Design review of the part built by this model. Coordinates are the model's own, in mm. Face numbers are marked on the shaded views. Coordinates: 2 decimals unless noted, no trailing zeros. Write each loop counter-clockwise with the first axis right and the second up, starting at its lowest first coordinate (ties: lowest second). Pieces come first, ordered by that corner, then holes.
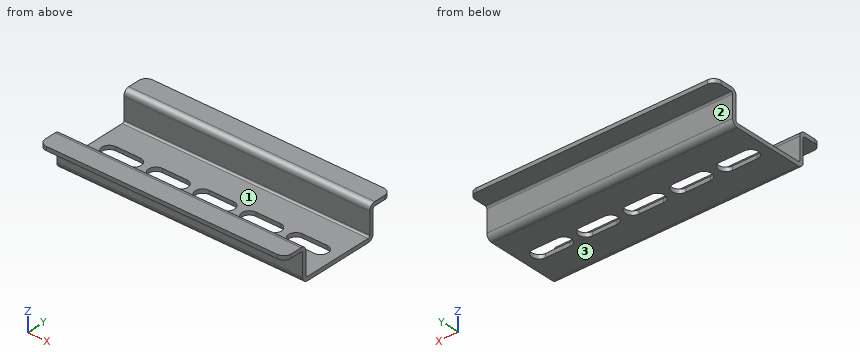
```python
from build123d import *

# Parameters (mm, degrees)
SKETCH_1_W                         = 100
SKETCH_1_H                         = 30
SM_BASE_FLANGE_1_DEPTH             = 1.6
SM_EDGE_FLANGE_1_STRIP_W           = 7.8732
SM_EDGE_FLANGE_1_STRIP_H           = 1.6
SM_EDGE_FLANGE_1_STRIP_CUT_DEPTH   = 100
SM_EDGE_FLANGE_1_STRIP_2_W         = 7.8732
SM_EDGE_FLANGE_1_STRIP_2_H         = 1.6
SM_EDGE_FLANGE_1_STRIP_CUT_2_DEPTH = 100
SM_EDGE_FLANGE_1_DEPTH             = 100
SM_EDGE_FLANGE_1_BEND_DEPTH        = 100
SM_EDGE_FLANGE_2_STRIP_W           = 7.8732
SM_EDGE_FLANGE_2_STRIP_H           = 1.6
SM_EDGE_FLANGE_2_STRIP_CUT_DEPTH   = 100
SM_EDGE_FLANGE_2_STRIP_2_W         = 7.8732
SM_EDGE_FLANGE_2_STRIP_2_H         = 1.6
SM_EDGE_FLANGE_2_STRIP_CUT_2_DEPTH = 100
SM_EDGE_FLANGE_2_DEPTH             = 100
SM_EDGE_FLANGE_2_BEND_DEPTH        = 100
CUT_EXTRUDE_1_DEPTH                = 58.175169436
CUT_EXTRUDE_2_DEPTH                = 58.532251825


# Sheet-metal steps are written as plain solids
with BuildPart() as part:
    # Sketch 1 → 基体-法兰1 (new body)
    with BuildSketch(Plane.XY):
        Rectangle(SKETCH_1_W, SKETCH_1_H)
    extrude(amount=-SM_BASE_FLANGE_1_DEPTH)

    # 边线-法兰1 strip (across the edge) → 边线-法兰1 strip cut (cut)
    with BuildSketch(Plane(origin=(50, 15, 0), x_dir=(0, -1, 0), z_dir=(-1, 0, 0))):
        with Locations((-3.2, -0.8)):
            Rectangle(SM_EDGE_FLANGE_1_STRIP_W, SM_EDGE_FLANGE_1_STRIP_H)
    extrude(amount=SM_EDGE_FLANGE_1_STRIP_CUT_DEPTH, mode=Mode.SUBTRACT)

    # 边线-法兰1 strip 2 (across the edge) → 边线-法兰1 strip cut 2 (cut)
    with BuildSketch(Plane(origin=(-50, -15, 0), x_dir=(0, 1, 0), z_dir=(1, 0, 0))):
        with Locations((-3.2, -0.8)):
            Rectangle(SM_EDGE_FLANGE_1_STRIP_2_W, SM_EDGE_FLANGE_1_STRIP_2_H)
    extrude(amount=SM_EDGE_FLANGE_1_STRIP_CUT_2_DEPTH, mode=Mode.SUBTRACT)

    # 边线-法兰1 section (across the edge) → 边线-法兰1 (add)
    with BuildSketch(Plane(origin=(50, 15, 0), x_dir=(0, -1, 0), z_dir=(-1, 0, 0))):
        with BuildLine():
            Line((-1.6, 0.7366), (-1.6, 10.4))
            Line((-1.6, 10.4), (0, 10.4))
            Line((0, 10.4), (0, 0.7366))
            ThreePointArc((0, 0.7366), (0.215745145, 0.215745145), (0.7366, 0))
            Line((0.7366, 0), (0.7366, -1.6))
            ThreePointArc((0.7366, -1.6), (-0.915625705, -0.915625705), (-1.6, 0.7366))
        make_face()
    extrude(amount=SM_EDGE_FLANGE_1_DEPTH)

    # 边线-法兰1 section 2 (across the edge) → 边线-法兰1 bend (add)
    with BuildSketch(Plane(origin=(-50, -15, 0), x_dir=(0, 1, 0), z_dir=(1, 0, 0))):
        with BuildLine():
            Line((-1.6, 0.7366), (-1.6, 10.4))
            Line((-1.6, 10.4), (0, 10.4))
            Line((0, 10.4), (0, 0.7366))
            ThreePointArc((0, 0.7366), (0.215745145, 0.215745145), (0.7366, 0))
            Line((0.7366, 0), (0.7366, -1.6))
            ThreePointArc((0.7366, -1.6), (-0.915625705, -0.915625705), (-1.6, 0.7366))
        make_face()
    extrude(amount=SM_EDGE_FLANGE_1_BEND_DEPTH)

    # 边线-法兰2 strip (across the edge) → 边线-法兰2 strip cut (cut)
    with BuildSketch(Plane(origin=(-50, 16.6, 10.4), x_dir=(0, 0, -1), z_dir=(1, 0, 0))):
        with Locations((-3.2, -0.8)):
            Rectangle(SM_EDGE_FLANGE_2_STRIP_W, SM_EDGE_FLANGE_2_STRIP_H)
    extrude(amount=SM_EDGE_FLANGE_2_STRIP_CUT_DEPTH, mode=Mode.SUBTRACT)

    # 边线-法兰2 strip 2 (across the edge) → 边线-法兰2 strip cut 2 (cut)
    with BuildSketch(Plane(origin=(50, -16.6, 10.4), x_dir=(0, 0, -1), z_dir=(-1, 0, 0))):
        with Locations((-3.2, -0.8)):
            Rectangle(SM_EDGE_FLANGE_2_STRIP_2_W, SM_EDGE_FLANGE_2_STRIP_2_H)
    extrude(amount=SM_EDGE_FLANGE_2_STRIP_CUT_2_DEPTH, mode=Mode.SUBTRACT)

    # 边线-法兰2 section (across the edge) → 边线-法兰2 (add)
    with BuildSketch(Plane(origin=(-50, 16.6, 10.4), x_dir=(0, 0, -1), z_dir=(1, 0, 0))):
        with BuildLine():
            Line((-1.6, 0.7366), (-1.6, 8.4))
            Line((-1.6, 8.4), (0, 8.4))
            Line((0, 8.4), (0, 0.7366))
            ThreePointArc((0, 0.7366), (0.215745145, 0.215745145), (0.7366, 0))
            Line((0.7366, 0), (0.7366, -1.6))
            ThreePointArc((0.7366, -1.6), (-0.915625705, -0.915625705), (-1.6, 0.7366))
        make_face()
    extrude(amount=SM_EDGE_FLANGE_2_DEPTH)

    # 边线-法兰2 section 2 (across the edge) → 边线-法兰2 bend (add)
    with BuildSketch(Plane(origin=(50, -16.6, 10.4), x_dir=(0, 0, -1), z_dir=(-1, 0, 0))):
        with BuildLine():
            Line((-1.6, 0.7366), (-1.6, 8.4))
            Line((-1.6, 8.4), (0, 8.4))
            Line((0, 8.4), (0, 0.7366))
            ThreePointArc((0, 0.7366), (0.215745145, 0.215745145), (0.7366, 0))
            Line((0.7366, 0), (0.7366, -1.6))
            ThreePointArc((0.7366, -1.6), (-0.915625705, -0.915625705), (-1.6, 0.7366))
        make_face()
    extrude(amount=SM_EDGE_FLANGE_2_BEND_DEPTH)

    # 草图18 → 切除-拉伸1 (cut, through all)
    with BuildSketch(Plane.XY):
        with BuildLine():
            Line((50, 25), (47, 25))
            ThreePointArc((47, 25), (49.121320344, 24.121320344), (50, 22))
            Line((50, 22), (50, 25))
        make_face()
        with BuildLine():
            Line((-47, 25), (-50, 25))
            Line((-50, 25), (-50, 22))
            ThreePointArc((-50, 22), (-49.121320344, 24.121320344), (-47, 25))
        make_face()
        with BuildLine():
            Line((-50, -22), (-50, -25))
            Line((-50, -25), (-47, -25))
            ThreePointArc((-47, -25), (-49.121320344, -24.121320344), (-50, -22))
        make_face()
        with BuildLine():
            Line((47, -25), (50, -25))
            Line((50, -25), (50, -22))
            ThreePointArc((50, -22), (49.121320344, -24.121320344), (47, -25))
        make_face()
    extrude(amount=CUT_EXTRUDE_1_DEPTH, mode=Mode.SUBTRACT)

    # 草图19 → 切除-拉伸2 (cut, through all)
    with BuildSketch(Plane(origin=(0, 0, -1.6), x_dir=(-1, 0, 0), z_dir=(0, 0, -1))):
        with BuildLine():
            Line((-43, 3), (-33, 3))
            ThreePointArc((-33, 3), (-30, 0), (-33, -3))
            Line((-33, -3), (-43, -3))
            ThreePointArc((-43, -3), (-46, 0), (-43, 3))
        make_face()
        with BuildLine():
            Line((-24, 3), (-14, 3))
            ThreePointArc((-14, 3), (-11, 0), (-14, -3))
            Line((-14, -3), (-24, -3))
            ThreePointArc((-24, -3), (-27, 0), (-24, 3))
        make_face()
        with BuildLine():
            Line((-5, 3), (5, 3))
            ThreePointArc((5, 3), (8, 0), (5, -3))
            Line((5, -3), (-5, -3))
            ThreePointArc((-5, -3), (-8, 0), (-5, 3))
        make_face()
        with BuildLine():
            Line((14, 3), (24, 3))
            ThreePointArc((24, 3), (27, 0), (24, -3))
            Line((24, -3), (14, -3))
            ThreePointArc((14, -3), (11, 0), (14, 3))
        make_face()
        with BuildLine():
            Line((33, 3), (43, 3))
            ThreePointArc((43, 3), (46, 0), (43, -3))
            Line((43, -3), (33, -3))
            ThreePointArc((33, -3), (30, 0), (33, 3))
        make_face()
    extrude(amount=-CUT_EXTRUDE_2_DEPTH, mode=Mode.SUBTRACT)


solid = part.part
```
(1) Consider section A-A (z = 5.5). Give the boundary of the cut face in (x, y).
(2) Wall thickness on line 1 (Y direction, x = -28, z = 4.25); line 2 (Z direction, x = -28.5, y = 22.5); line 3 (Z direction, x = -4, y = -8): over which ranges is each line inside the solid? List them lowest first.
(3) Consider section C-C (y = -2). Give the boundary of the cut face in (x, z).
(4) Consider section D-D (y = -7.5). Give the boundary of the cut face in (x, z).
(5) Consider section B-B (x = -36). Give the boundary of the cut face in (y, z).
(6) Insertion check: pin 1 Ø0.8 at (x, z) = (-36.5, -0.5) entering from -Y; pin 2 Ø0.8 at (x, z) = (-36.5, -1) entering from +Y; pin 3 Ø5 at (x, y) = (20.5, -12) entering from +Z; pin 4 Ø1.5 at (y, z) = (3.5, 1) entering from -X. Each pin has a flat end and moves straight along its axis. Give the tip position at first contact, or say it passes through.
(7) Mouldability with a two-part tool opening along Y and no side actions: class the marked faces 1, 2 and 3 as +Y half, -Y half, draft (parallel to the pull), parting line (faces both ways), or undercut.
Results:
1. outline: (-50, -16.6) - (50, -16.6) - (50, -15) - (-50, -15) - close; (-50, 15) - (50, 15) - (50, 16.6) - (-50, 16.6) - close
2. line 1: y = -16.6 to -15, 15 to 16.6
2. line 2: z = 10.4 to 12
2. line 3: z = -1.6 to 0
3. outline: (-50, -1.6) - (-45.24, -1.6) - (-45.24, 0) - (-50, 0) - close; (-30.76, -1.6) - (-26.24, -1.6) - (-26.24, 0) - (-30.76, 0) - close; (-11.76, -1.6) - (-7.24, -1.6) - (-7.24, 0) - (-11.76, 0) - close; (7.24, -1.6) - (11.76, -1.6) - (11.76, 0) - (7.24, 0) - close; (26.24, -1.6) - (30.76, -1.6) - (30.76, 0) - (26.24, 0) - close; (45.24, -1.6) - (50, -1.6) - (50, 0) - (45.24, 0) - close
4. outline: (-50, -1.6) - (50, -1.6) - (50, 0) - (-50, 0) - close
5. outline: (-25, 10.4) - (-17.34, 10.4) arc R0.74 cw to (-16.6, 9.66) - (-16.6, 0.74) arc R2.34 ccw to (-14.26, -1.6) - (-3, -1.6) - (-3, 0) - (-14.26, 0) arc R0.74 cw to (-15, 0.74) - (-15, 9.66) arc R2.34 ccw to (-17.34, 12) - (-25, 12) - close; (3, -1.6) - (14.26, -1.6) arc R2.34 ccw to (16.6, 0.74) - (16.6, 9.66) arc R0.74 cw to (17.34, 10.4) - (25, 10.4) - (25, 12) - (17.34, 12) arc R2.34 ccw to (15, 9.66) - (15, 0.74) arc R0.74 cw to (14.26, 0) - (3, 0) - close
6. pin 1: stops at y = -16.45
6. pin 2: stops at y = 16.18
6. pin 3: stops at z = 0.04
6. pin 4: passes through
7. face 1: undercut
7. face 2: +Y half
7. face 3: draft
